from build123d import *

# Parameters (mm, degrees)
SKETCH_R        = 3
PAD_DEPTH       = 6.5
SKETCH001_R     = 6.1
SKETCH001_R_2   = 3
PAD001_DEPTH    = 10
PAD002_DEPTH    = 13
SKETCH003_R     = 6.1
POCKET_DEPTH    = 6
POCKET001_DEPTH = 6.5
SKETCH005_R     = 2.1
POCKET002_DEPTH = 4.201


with BuildPart() as part:
    # Sketch → Pad (new body)
    with BuildSketch(Plane.XY):
        Polygon((9.814955, 0), (4.907477, 8.5), (-4.907477, 8.5), (-9.814955, 0), (-4.907477, -8.5), (4.907477, -8.5), align=None)
        Circle(SKETCH_R, mode=Mode.SUBTRACT)
    extrude(amount=PAD_DEPTH)

    # Sketch001 (on Face9 of Pad) → Pad001 (join)
    with BuildSketch(Plane.XY.offset(6.5)):
        Circle(SKETCH001_R)
        Circle(SKETCH001_R_2, mode=Mode.SUBTRACT)
    extrude(amount=PAD001_DEPTH)

    # Sketch002 (on Face12 of Pad001) → Pad002 (join)
    with BuildSketch(Plane.XY.offset(16.5)):
        with BuildLine():
            Line((-1.658312, 2.5), (1.658312, 2.5))
            ThreePointArc((1.658312, 2.5), (0, 3), (-1.658312, 2.5))
        make_face()
    extrude(amount=-PAD002_DEPTH)

    # Sketch003 (on Face15 of Pad002) → Pocket (cut)
    with BuildSketch(Plane.XY.offset(16.5)):
        Circle(SKETCH003_R)
    extrude(amount=-POCKET_DEPTH, mode=Mode.SUBTRACT)

    # Sketch004 (on Face4 of Pocket) → Pocket001 (cut)
    with BuildSketch(Plane(origin=(0, 0, 0), x_dir=(1, 0, 0), z_dir=(0, 0, -1))):
        with BuildLine():
            ThreePointArc((2.5, -2.727636), (0, 3.7), (-2.5, -2.727636))
            Line((-2.5, -4.3), (-2.5, -2.727636))
            Line((2.5, -4.3), (-2.5, -4.3))
            Line((2.5, -4.3), (2.5, -2.727636))
        make_face()
    extrude(amount=-POCKET001_DEPTH, mode=Mode.SUBTRACT)

    # Sketch005 (on Face9 of Pocket001) → Pocket002 (cut, through all)
    with BuildSketch(Plane.XZ.offset(-4.3)):
        with Locations((0, 3.4)):
            Circle(SKETCH005_R)
    extrude(amount=-POCKET002_DEPTH, mode=Mode.SUBTRACT)


solid = part.part
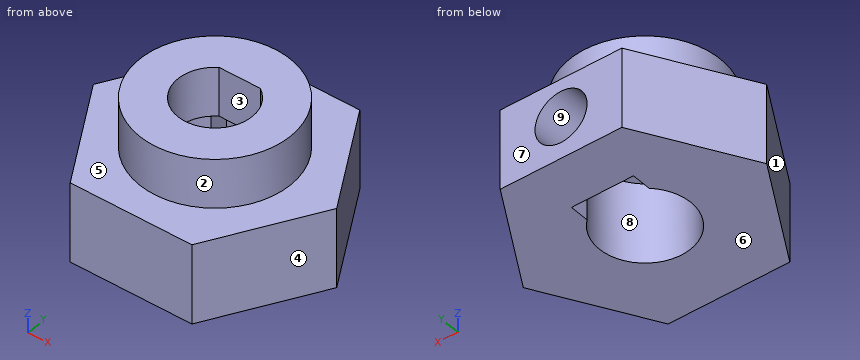
Here's how the part is built. I have some questions about the finished solid (model axes, mm). Face numbers are marked on the shaded views. A direction names the side the tool comes from. Coordinates: 2 decimals unless noted, no trailing zeros. Order: outer loops, then holes, each group sorted by start corner. A loop starts at its lowest first (then second) coordinate and runs counter-clockwise, first axis right, second up.
Item 1: For the marked faces 5, 6, 7, 8 and 9, which set-ups out of +Z, -Z, +X, -X, +Y, -Y let a thin tool reach every point of the face, with its end or its side?
Result sheet:
face 5: +Z
face 6: -Z, +X, -X, +Y, -Y
face 7: +Z, -Z, +X, -X, +Y
face 8: -Z
face 9: +Y
Item 2: If we section it at B-B on x = 0: List the corners of the cut face in (y, z) for me, plus the area to 3 significant figures.
Result sheet:
outline: (-8.5, 0) - (-3.7, 0) - (-3.7, 6.5) - (-3, 6.5) - (-3, 10.5) - (-6.1, 10.5) - (-6.1, 6.5) - (-8.5, 6.5) - close; (2.5, 6.5) - (4.3, 6.5) - (4.3, 5.5) - (8.5, 5.5) - (8.5, 6.5) - (6.1, 6.5) - (6.1, 10.5) - (2.5, 10.5) - close; (4.3, 0) - (8.5, 0) - (8.5, 1.3) - (4.3, 1.3) - close
area: 67.7 mm2
Item 3: If we section it at D-D on x = -5.75: List the corners of the cut face in (y, z) for me, plus the area to 3 significant figures.
Result sheet:
outline: (-7.04, 0) - (7.04, 0) - (7.04, 6.5) - (2.04, 6.5) - (2.04, 10.5) - (-2.04, 10.5) - (-2.04, 6.5) - (-7.04, 6.5) - close
area: 108 mm2
Item 4: If we section it at C-C on z = 3.4: List the corners of the cut face in (x, y) for me.
Result sheet:
outline: (-9.81, 0) - (-4.91, -8.5) - (4.91, -8.5) - (9.81, 0) - (4.91, 8.5) - (2.1, 8.5) - (2.1, 4.3) - (2.5, 4.3) - (2.5, 2.73) arc R3.7 cw (long way) to (-2.5, 2.73) - (-2.5, 4.3) - (-2.1, 4.3) - (-2.1, 8.5) - (-4.91, 8.5) - close
Item 5: For P1, Ø1.3, axis at y = 3.5, z = 2, coming from the +X side; P2, Ø0.8, axis at y = 3.5, z = 1.5, coming from the -X side; P3, Ø4, axis at y = 1.5, z = 8, coming from the +X side, each with a flat end and sliding along its axis, tell me the tip position at first contact or that it passes through.
Result sheet:
P1: stops at x = 8.17
P2: stops at x = -8.03
P3: stops at x = 9.71
Item 6: I need wall thicknesses on line 1 (Z direction, x = 0, y = 6.3); line 2 (Z direction, x = 0, y = 5.3); line 3 (Z direction, x = -5.75, y = 6). Which ranges of each line are inside material? Lowest first, please.
Result sheet:
line 1: z = 0 to 1.3, 5.5 to 6.5
line 2: z = 0 to 1.3, 5.5 to 10.5
line 3: z = 0 to 6.5
Item 7: If we section it at A-A on z = 6: List the corners of the cut face in (x, y) for me.
Result sheet:
outline: (-9.81, 0) - (-4.91, -8.5) - (4.91, -8.5) - (9.81, 0) - (4.91, 8.5) - (-4.91, 8.5) - close; hole (-2.5, 2.73) arc R3.7 ccw (long way) to (2.5, 2.73) - (2.5, 4.3) - (-2.5, 4.3) - close
Item 8: If we mould it in two halves opening along X, with no side actions, what happens to the marked faces 1, 2, 3 and 4? For each: +X half, -X half, draft (parallel to the pull), parting line (faces both ways), or undercut.
Result sheet:
face 1: -X half
face 2: parting line
face 3: undercut
face 4: +X half
